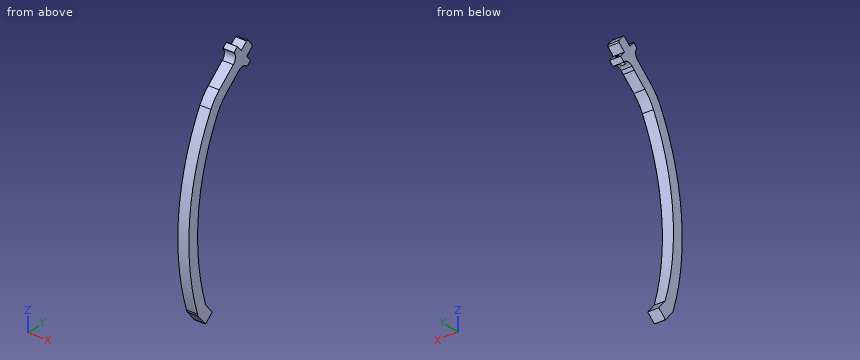
from build123d import *

# Parameters (mm, degrees)
AUFSATZ_LINEAR_AUSTRAGEN1_DEPTH  = 12
AUFSATZ_LINEAR_AUSTRAGEN3_DEPTH  = 12
AUFSATZ_LINEAR_AUSTRAGEN4_DEPTH  = 12
SCHNITT_LINEAR_AUSTRAGEN1_DEPTH  = 254.175024926
VERRUNDUNG1_R                    = 50
SKIZZE9_W                        = 12
SKIZZE9_H                        = 12
AUFSATZ_LINEAR_AUSTRAGEN6_DEPTH  = 11
AUFSATZ_LINEAR_AUSTRAGEN7_DEPTH  = 12
SKIZZE11_R                       = 1.75
SCHNITT_LINEAR_AUSTRAGEN3_DEPTH  = 10
SKIZZE12_R                       = 2.75
SCHNITT_LINEAR_AUSTRAGEN4_DEPTH  = 3.6
FASE1_SIZE                       = 1.5
SCHNITT_LINEAR_AUSTRAGEN8_DEPTH  = 254.549622303
SKIZZE11_3_R                     = 1.45
SCHNITT_LINEAR_AUSTRAGEN10_DEPTH = 6


with BuildPart() as part:
    # Skizze1 → Aufsatz-Linear austragen1 (new body)
    with BuildSketch(Plane(origin=(0, 0, 0), x_dir=(0, 0, -1), z_dir=(1, 0, 0))):
        with BuildLine():
            Line((-240, 65), (-230.735708163, 72.773663864))
            ThreePointArc((-230.735708163, 72.773663864), (-123.944567763, 17.242039243), (-3.735818811, 23.403668612))
            Line((-3.735818811, 23.403668612), (0, 12))
            ThreePointArc((0, 12), (-127.247502729, 5.681119716), (-240, 65))
        make_face()
    extrude(amount=AUFSATZ_LINEAR_AUSTRAGEN1_DEPTH)

    # Skizze4 → Aufsatz-Linear austragen3 (add)
    with BuildSketch(Plane(origin=(0, 0, 0), x_dir=(0, 0, -1), z_dir=(1, 0, 0))):
        with BuildLine():
            Line((-3.735818811, 23.403668612), (6.769031275, 32.218284445))
            Line((6.769031275, 32.218284445), (14.482482591, 23.025751128))
            Line((14.482482591, 23.025751128), (2.225771501, 12.741149373))
            ThreePointArc((2.225771501, 12.741149373), (1.113785782, 12.367871772), (0, 12))
            Line((0, 12), (-3.735818811, 23.403668612))
        make_face()
    extrude(amount=AUFSATZ_LINEAR_AUSTRAGEN3_DEPTH)

    # Skizze5 → Aufsatz-Linear austragen4 (add)
    with BuildSketch(Plane(origin=(12, 0, 0), x_dir=(0, 0, -1), z_dir=(1, 0, 0))):
        Polygon((-231.662517154, 71.995978781), (-222.469983836, 79.709430098), (-210.899806862, 65.920630121), (-192.948331238, 44.526894555), (-220.092340179, 58.207178805), align=None)
    extrude(amount=-AUFSATZ_LINEAR_AUSTRAGEN4_DEPTH)

    # Skizze6 → Schnitt-Linear austragen1 (cut, through all)
    with BuildSketch(Plane(origin=(12, 0, 0), x_dir=(0, 0, -1), z_dir=(1, 0, 0))):
        Polygon((-231.662517154, 71.995978781), (-199.510648028, 33.678873242), (-204.367668784, 29.603348917), (-240, 65), align=None)
    extrude(amount=-SCHNITT_LINEAR_AUSTRAGEN1_DEPTH, mode=Mode.SUBTRACT)

    # Verrundung1
    verrundung1_edges = [part.edges().sort_by_distance(p)[0] for p in [
        (6, 44.526894555, 192.948331238),
        (6, 35.285406895, 200.858689823),
    ]]
    fillet(verrundung1_edges, radius=VERRUNDUNG1_R)

    # Skizze9 → Aufsatz-Linear austragen6 (add)
    with BuildSketch(Plane(origin=(0, 156.320496136, 131.168470653), x_dir=(1, 0, 0), z_dir=(0, 0.7660444431189836, 0.6427876096865328))):
        with Locations((6, -125.185660837)):
            Rectangle(SKIZZE9_W, SKIZZE9_H)
    extrude(amount=AUFSATZ_LINEAR_AUSTRAGEN6_DEPTH)

    # Skizze10 → Aufsatz-Linear austragen7 (add)
    with BuildSketch(Plane.ZY):
        with BuildLine():
            Line((231.662517154, 71.995978781), (237.790872699, 66.853677904))
            Line((237.790872699, 66.853677904), (233.93414704, 62.257411245))
            ThreePointArc((233.93414704, 62.257411245), (228.094600221, 64.098613285), (222.663490618, 61.271356578))
            Line((222.663490618, 61.271356578), (231.662517154, 71.995978781))
        make_face()
        with BuildLine():
            Line((213.470957301, 68.984807894), (222.469983836, 79.709430098))
            Line((222.469983836, 79.709430098), (216.341628291, 84.851730975))
            Line((216.341628291, 84.851730975), (212.484902633, 80.255464316))
            ThreePointArc((212.484902633, 80.255464316), (215.31215934, 74.824354713), (213.470957301, 68.984807894))
        make_face()
    extrude(amount=-AUFSATZ_LINEAR_AUSTRAGEN7_DEPTH)

    # Skizze11 → Schnitt-Linear austragen3 (cut)
    with BuildSketch(Plane(origin=(0, 156.320496136, 131.168470653), x_dir=(1, 0, 0), z_dir=(0, 0.7660444431189826, 0.642787609686534))):
        with Locations(Location((6, -115.785660837, 0), (0, 0, 270))):
            Circle(SKIZZE11_R)
    extrude(amount=-SCHNITT_LINEAR_AUSTRAGEN3_DEPTH, mode=Mode.SUBTRACT)

    # Skizze12 → Schnitt-Linear austragen4 (cut)
    with BuildSketch(Plane(origin=(0, 148.660051704, 124.740594556), x_dir=(1, 0, 0), z_dir=(0, 0.7660444431189826, 0.642787609686534))):
        with Locations((6, -115.785660837)):
            Circle(SKIZZE12_R)
    extrude(amount=SCHNITT_LINEAR_AUSTRAGEN4_DEPTH, mode=Mode.SUBTRACT)

    # Fase1
    fase1_edges = [part.edges().sort_by_distance(p)[0] for p in [
        (6, 88.135918972, 229.540647543),
        (6, 80.422467656, 238.73318086),
    ]]
    chamfer(fase1_edges, length=FASE1_SIZE)

    # Skizze16 → Schnitt-Linear austragen8 (cut, through all)
    with BuildSketch(Plane(origin=(12, 0, 0), x_dir=(0, 0, -1), z_dir=(1, 0, 0))):
        Polygon((-222.469983836, 79.709430098), (-222.546588281, 79.645151337), (-228.717349334, 86.999177991), (-228.640744889, 87.063456752), align=None)
        Polygon((-237.833278207, 79.350005435), (-231.662517154, 71.995978781), (-231.585912709, 72.060257542), (-237.756673762, 79.414284196), align=None)
    extrude(amount=-SCHNITT_LINEAR_AUSTRAGEN8_DEPTH, mode=Mode.SUBTRACT)

    # Skizze11<3> → Schnitt-Linear austragen10 (cut)
    with BuildSketch(Plane(origin=(0, 156.320496136, 131.168470653), x_dir=(1, 0, 0), z_dir=(0, 0.7660444431189826, 0.642787609686534))):
        with Locations(Location((6, -134.585660837, 0), (0, 0, 270))):
            Circle(SKIZZE11_3_R)
    extrude(amount=-SCHNITT_LINEAR_AUSTRAGEN10_DEPTH, mode=Mode.SUBTRACT)


solid = part.part
Part model, mm, in its own coordinate system. Coordinates: 2 decimals unless noted, no trailing zeros. Order: outer loops, then holes, each group sorted by start corner. A loop starts at its lowest first (then second) coordinate and runs counter-clockwise, first axis right, second up. Notation, with made-up numbers: M 27.25,25 L 82.25,25 A21 ccw 82.25,32 Z; hole C 89,13 d4. An arc over 180 degrees is marked long. One line per question, with ' | ' between items.
Q1. Drill centre lines: line 1 (Z direction, x = 7.5, y = 63); line 2 (Z direction, x = 9, y = 62.5); line 3 (Z direction, x = 11.75, y = 57). Where is each one in solid material? Low to high.
A:
line 1: z = 208.45 to 224.69, 232.89 to 234.56 | line 2: z = 208.03 to 223.95, 233.63 to 234.14 | line 3: z = 203.41 to 219.08
Q2. Slice it at B-B (z = 77). Give the cut face in (x, y).
A:
outline: M 0,0.01 L 12,0.01 L 12,12.01 L 0,12.01 Z
Q3. Slice it at C-C (y = 45). Give the cut face in (x, z).
A:
outline: M 0,192.27 L 12,192.27 L 12,209.01 L 0,209.01 Z
Q4. Slice it at A-A (y = 20). Give the cut face in (x, z), and give its area (3 significant figures).
A:
outline: M 0,-10.88 L 12,-10.88 L 12,15.11 L 0,15.11 Z; M 0,135.24 L 12,135.24 L 12,171.4 L 0,171.4 Z | area: 746 mm^2
Q5. Pin check, flat tips, straight feed: P1, Ø1, axis at x = 10, z = 146.5, coming from the -Y side; P2, Ø5, axis at x = 8, y = 75.5, coming from the -Z side. Stop position of each tip, or through.
A:
P1: stops at y = 10.62 | P2: stops at z = 214.34
